Here's the drawing with two shaded views (mm, measured from the low corner). I have some questions. Give positions to 0.01 mm unless a question says otherwise; leave off trailing zeros. Order: outer loops, then holes, each group sorted by start corner. A loop starts at its lowest first (then second) coordinate and runs counter-clockwise, first axis right, second up. Notation, with made-up numbers: M 43,13 L 84,13 A20 ccw 84,45 Z; hole C 1,37 d9. An arc over 180 degrees is marked long. One line per question, with ' | ' between items. Start each with the question number.
1) If we section it at C-C, the plane x = 12: Please give me the cut outline in (y, z), plus the area to 3 significant figures.
2) If we section it at A-A, the plane x = 2: Please give me the cut outline in (y, z).
3) Please list where these lines run through material, in increasing order: line 1 along Y through (x, z) = (14.25, 20.75); line 2 along X through (y, z) = (30, 16.25); line 3 along X through (y, z) = (8.5, 13.5). Write a range as [from, to].
4) I'm going to push flat-ended pins straight in: pin 1 Ø10 at (y, z) = (52, 13.5) entering from -X; pin 2 Ø8 at (y, z) = (25.5, 17.5) entering from +X; pin 3 Ø1.5 at (y, z) = (16, 11) entering from +X. Where does each tip first touch, or does it pass through?
5) If we section it at D-D, the plane y = 34.5: Please give me the cut outline in (x, z), plus the area to 3 significant figures.
6) Thinking about a two-plate mould opening in Y: for the marked faces 1, 2 and 3, which applies, +Y half, -Y half, draft (parallel to the pull), parting line (faces both ways), or undercut?
7) If we section it at B-B, the plane z = 12: Please give me the cut outline in (x, y), plus the area to 3 significant figures.
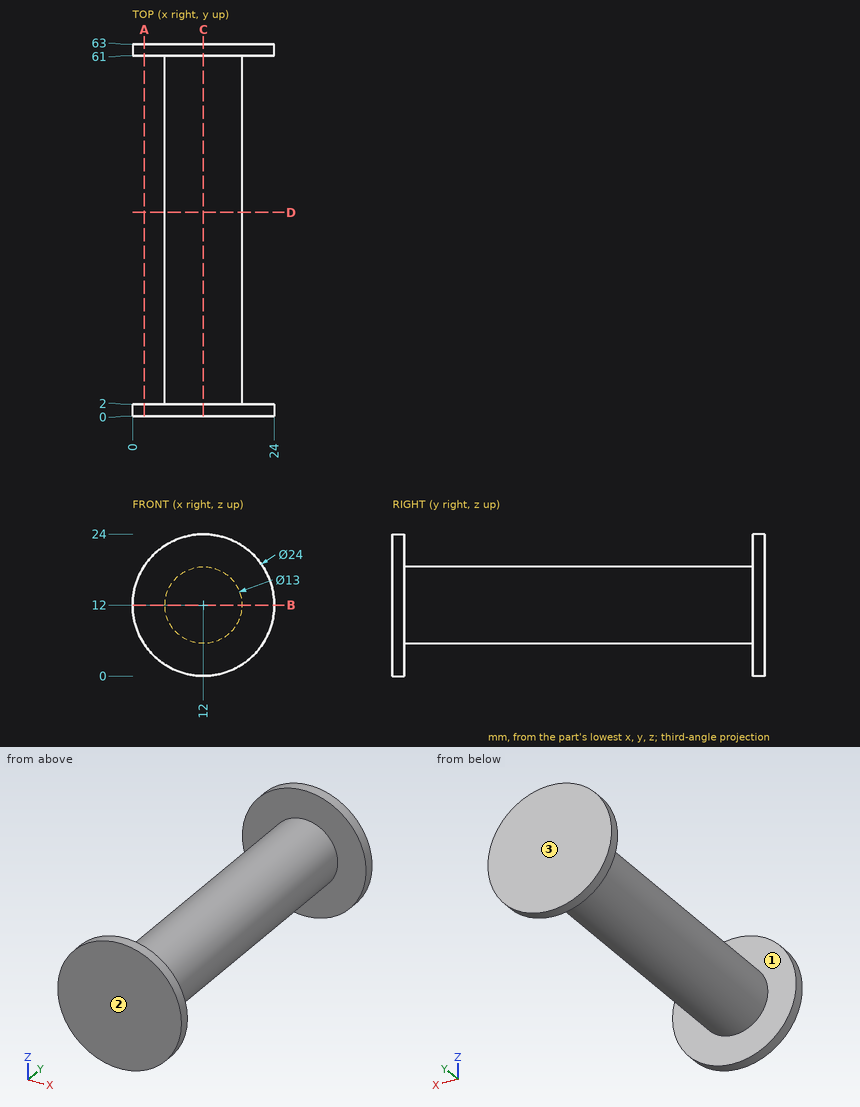
Results found:
1) outline: M 0,0 L 2,0 L 2,5.5 L 61,5.5 L 61,0 L 63,0 L 63,24 L 61,24 L 61,18.5 L 2,18.5 L 2,24 L 0,24 Z | area: 863 mm²
2) outline: M 0,5.37 L 2,5.37 L 2,18.63 L 0,18.63 Z; M 61,5.37 L 63,5.37 L 63,18.63 L 61,18.63 Z
3) line 1: y = [0, 2], [61, 63] | line 2: x = [7.08, 16.92] | line 3: x = [5.68, 18.32]
4) pin 1: stops at x = 5.5 | pin 2: stops at x = 18.32 | pin 3: stops at x = 18.5
5) outline: C 12,12 d13 | area: 133 mm²
6) face 1: undercut | face 2: -Y half | face 3: +Y half
7) outline: M 0,0 L 24,0 L 24,2 L 18.5,2 L 18.5,61 L 24,61 L 24,63 L 0,63 L 0,61 L 5.5,61 L 5.5,2 L 0,2 Z | area: 863 mm²
